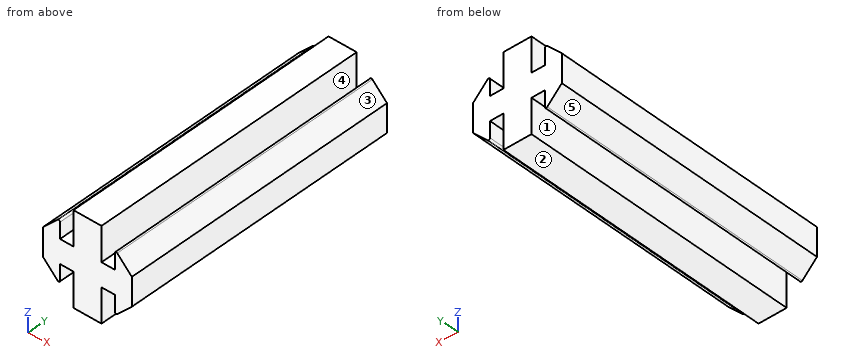
Autodesk Inventor part; units mm, degrees
ref_plane "YZ Plane" through (0, 0, 0) normal (1, 0, 0) x (0, 1, 0)
ref_plane "XZ Plane" through (0, 0, 0) normal (0, 1, 0) x (-1, 0, 0)
ref_plane "XY Plane" through (0, 0, 0) normal (0, 0, 1) x (1, 0, 0)
sketch "Sketch1" plane through (0, 0, 0) normal (0, 1, 0) x (-1, 0, 0)
  line L0 (0, 0) -> (5.08, 0)
  line L1 (5.08, 0) -> (5.08, -16.637)
  line L2 (5.08, -16.637) -> (0, -16.637)
  line L3 (0, -16.637) -> (0, 0)
  line L4 (0, -6.1892) -> (7.493, -6.1892)
  line L5 (7.493, -6.1892) -> (7.493, -10.4478)
  line L6 (7.493, -10.4478) -> (0, -10.4478)
  line L7 (10.5664, -5.7785) -> (10.5664, -10.8585)
  line L8 (7.493, -13.9319) -> (7.493, -2.7051)
  line L9 (7.493, -13.9319) -> (10.5664, -10.8585)
  line L10 (7.493, -2.7051) -> (10.5664, -5.7785)
  line L11 (0, -6.1892) -> (-2.413, -6.1892)
  line L12 (-2.413, -10.4478) -> (0, -10.4478)
  line L13 (-5.4864, -5.7785) -> (-5.4864, -10.8585)
  line L14 (-2.413, -13.9319) -> (-2.413, -2.7051)
  line L15 (-2.413, -13.9319) -> (-5.4864, -10.8585)
  line L16 (-2.413, -2.7051) -> (-5.4864, -5.7785)
  point P0 (-4.9276, -6.1892)
  dimension "d0" = 5.08
  dimension "d1" = 16.637
  dimension "d2" = 2.413
  dimension "d9" = 3.0734
  dimension "d12" = 0
  dimension "d16" = 11.2268
  dimension "d20" = 135
  dimension "d21" = 135
  dimension "d24" = 6.1893
  dimension "d25" = 16.637
  dimension "d26" = 3.4842
  dimension "d33" = 3.4842
  dimension "d34" = 3.0734
  dimension "d35" = 2.413
  dimension "d36" = 6.1893
  dimension "d37" = 5.08
  dimension "d38" = 5.08
  dimension "d39" = 135
  dimension "d40" = 135
extrude "Extrusion2" add sketch "Sketch1" along normal blind 50.8
fillet "Fillet1" radius 0.254 4 edges at (2.413, 25.4, -13.9319) (-7.493, 25.4, -13.9319) (2.413, 25.4, -2.7051) (-7.493, 25.4, -2.7051)
equation "\"d16\" = d15"
equation "\"d21\" = d20"
equation "\"d24\" = -0.5 * d4 + 0.5 * d25"
properties part number "20X20 lift conecter" material "PC/ABS Plastic"
Geometry check sheet. Reference: the model listing, model coordinates, mm. Face numbers are marked on the shaded views. A direction names the side the tool comes from. Coordinates: 2 decimals unless noted, no trailing zeros. Order: outer loops, then holes, each group sorted by start corner. A loop starts at its lowest first (then second) coordinate and runs counter-clockwise, first axis right, second up. Notation, with made-up numbers: M -23.5,42 L -0.5,42 A25 cw -0.5,57 Z; hole C 16,4.5 d8. An arc over 180 degrees is marked long. One line per question, with ' | ' between items. Start each with the question number.
Item 1: Cross-section at B-B on z = -4.5. Enter the section's corners in (x, y), then the cut area to 3 significant figures.
Item 2: Draft check along X on the marked faces 3, 4 and 5. Enter one of: pulls with the +X half, pulls with the -X half, needs draft (parallel to the pull), parting line crosses it, or undercut.
Item 3: Set-up check for the marked faces 1 and 2: record each of +Z, -Z, +X, -X, +Y, -Y from which the full face is reachable in a straight line by a thin tool's end or side.
Item 4: Cross-section at A-A on y = 38.5. Enter the section's corners in (x, z), then the cut area to 3 significant figures.
Item 5: Cross-section at D-D on z = -2. Enter the section's corners in (x, y), then the cut area to 3 significant figures.
Item 6: Material ranges on L1, parallel to X at y = 37.5, z = -10.5; L2, parallel to X at y = 37.5, z = -12.5; L3, parallel to X at y = 22, z = -1.25, recorded low to high. Write a range as [from, to].
Item 7: Gauge pin test, flat ends, axial feed: pin 1 (3 mm diameter, centred on y = 35.5, z = -12.5, fed in from +X); pin 2 (7 mm diameter, centred on y = 22.5, z = -14.5, fed in from -X); pin 3 (1.4 mm diameter, centred on y = 32.5, z = -5, fed in from -X). Record the tip position at first contact, or that the pin passes through.
Item 8: Cross-section at C-C on x = 1.5. Enter the section's corners in (y, z), then the cut area to 3 significant figures.
Findings:
1) outline: M -9.29,0 L -7.49,0 L -7.49,50.8 L -9.29,50.8 Z; M -5.08,0 L 0,0 L 0,50.8 L -5.08,50.8 Z; M 2.41,0 L 4.21,0 L 4.21,50.8 L 2.41,50.8 Z | area: 440 mm²
2) face 3: pulls with the +X half | face 4: undercut | face 5: pulls with the -X half
3) face 1: -Z, +Y, -Y | face 2: -Z, +X, -X, +Y, -Y
4) outline: M -10.57,-10.86 L -7.93,-13.5 A0.25 ccw -7.49,-13.32 L -7.49,-10.45 L -5.08,-10.45 L -5.08,-16.64 L 0,-16.64 L 0,-10.45 L 2.41,-10.45 L 2.41,-13.32 A0.25 ccw 2.85,-13.5 L 5.49,-10.86 L 5.49,-5.78 L 2.85,-3.14 A0.25 ccw 2.41,-3.32 L 2.41,-6.19 L 0,-6.19 L 0,0 L -5.08,0 L -5.08,-6.19 L -7.49,-6.19 L -7.49,-3.32 A0.25 ccw -7.93,-3.14 L -10.57,-5.78 Z | area: 155 mm²
5) outline: M -5.08,0 L 0,0 L 0,50.8 L -5.08,50.8 Z | area: 258 mm²
6) L1: x = [-10.57, -7.49], [-5.08, 0], [2.41, 5.49] | L2: x = [-8.92, -7.49], [-5.08, 0], [2.41, 3.84] | L3: x = [-5.08, 0]
7) pin 1: stops at x = 5.34 | pin 2: stops at x = -10.42 | pin 3: stops at x = -10.49
8) outline: M 0,-10.45 L 50.8,-10.45 L 50.8,-6.19 L 0,-6.19 Z | area: 216 mm²
